```python
from build123d import *

# Parameters (mm, degrees)
SKETCH1_W           = 31.25
SKETCH1_H           = 36.32
SKETCH1_R           = 1.5
BOSS_EXTRUDE2_DEPTH = 2
FILLET1_R           = 2
BOSS_EXTRUDE3_DEPTH = 6


with BuildPart() as part:
    # Sketch1 → Boss-Extrude2 (new body)
    with BuildSketch(Plane(origin=(0, 0, 0), x_dir=(1, 0, 0), z_dir=(0, 1, 0))):
        with Locations((-0.273367395, -0.136683698)):
            Rectangle(SKETCH1_W, SKETCH1_H)
        with Locations((-0.273367395, 14.023316302)):
            Circle(SKETCH1_R, mode=Mode.SUBTRACT)
        with Locations((-11.898367395, -0.136683698)):
            Circle(SKETCH1_R, mode=Mode.SUBTRACT)
        with Locations((-0.273367395, -14.296683698)):
            Circle(SKETCH1_R, mode=Mode.SUBTRACT)
        with Locations((11.351632605, -0.136683698)):
            Circle(SKETCH1_R, mode=Mode.SUBTRACT)
    extrude(amount=BOSS_EXTRUDE2_DEPTH)

    # Fillet1
    fillet1_edges = [part.edges().sort_by_distance(p)[0] for p in [
        (15.351632605, 1, 18.296683698),
        (-15.898367395, 1, 18.296683698),
        (-15.898367395, 1, -18.023316302),
        (15.351632605, 1, -18.023316302),
    ]]
    fillet(fillet1_edges, radius=FILLET1_R)

    # Sketch3 → Boss-Extrude3 (add)
    with BuildSketch(Plane(origin=(0, 2, 0), x_dir=(1, 0, 0), z_dir=(0, 1, 0))):
        with BuildLine():
            Line((13.351632605, 19.523316302), (-13.898367395, 19.523316302))
            ThreePointArc((-13.898367395, 19.523316302), (-16.373241129, 18.498190037), (-17.398367395, 16.023316302))
            Line((-17.398367395, 16.023316302), (-17.398367395, -16.296683698))
            ThreePointArc((-17.398367395, -16.296683698), (-16.373241129, -18.771557432), (-13.898367395, -19.796683698))
            Line((-13.898367395, -19.796683698), (13.351632605, -19.796683698))
            ThreePointArc((13.351632605, -19.796683698), (15.826506339, -18.771557432), (16.851632605, -16.296683698))
            Line((16.851632605, -16.296683698), (16.851632605, 16.023316302))
            ThreePointArc((16.851632605, 16.023316302), (15.826506339, 18.498190037), (13.351632605, 19.523316302))
        make_face()
        with BuildLine():
            Line((13.351632605, 18.023316302), (-13.898367395, 18.023316302))
            ThreePointArc((-13.898367395, 18.023316302), (-15.312580957, 17.437529865), (-15.898367395, 16.023316302))
            Line((-15.898367395, 16.023316302), (-15.898367395, -16.296683698))
            ThreePointArc((-15.898367395, -16.296683698), (-15.312580957, -17.71089726), (-13.898367395, -18.296683698))
            Line((-13.898367395, -18.296683698), (13.351632605, -18.296683698))
            ThreePointArc((13.351632605, -18.296683698), (14.765846167, -17.71089726), (15.351632605, -16.296683698))
            Line((15.351632605, -16.296683698), (15.351632605, 16.023316302))
            ThreePointArc((15.351632605, 16.023316302), (14.765846167, 17.437529865), (13.351632605, 18.023316302))
        make_face(mode=Mode.SUBTRACT)
    extrude(amount=-BOSS_EXTRUDE3_DEPTH)


solid = part.part
```
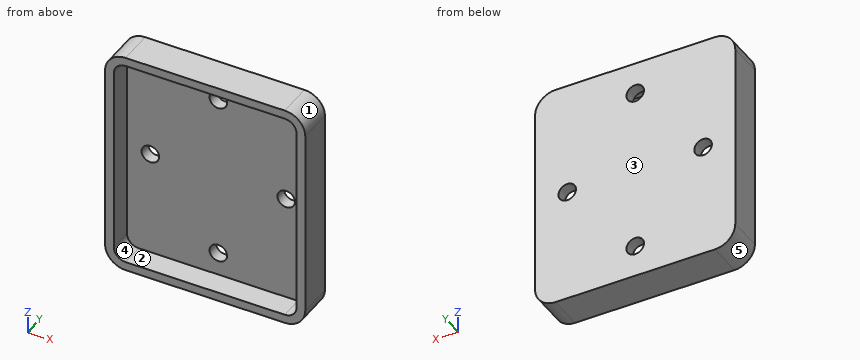
Geometry check sheet. Reference: the model listing, model coordinates, mm. Face numbers are marked on the shaded views. A direction names the side the tool comes from. Coordinates: 2 decimals unless noted, no trailing zeros. Order: outer loops, then holes, each group sorted by start corner. A loop starts at its lowest first (then second) coordinate and runs counter-clockwise, first axis right, second up. Notation, with made-up numbers: (66.5, 5.5) - (92.5, 5.5) arc R34 cw to (92.5, 42.5) - close; hole circle Ø6 at (87.5, -36). An arc over 180 degrees is marked (long way). Answer in a Markdown table with one row per item. Add a question column.
1. Draft check along Z on the marked faces 3, 4 and 5. Enter one of: +Z half, -Z half, draft (parallel to the pull), parting line (faces both ways), or undercut.
2. Access from +Z, -Z, +X, -X, +Y, -Y to the whole of each face (thin tool, end or side, straight path). Record for the marked faces 1 and 2.
3. Section check D-D (x = 0.5). Enter the section's corners in (y, z).
4. Section check C-C (x = -8.5). Enter the section's corners in (y, z), plus the area to 3 significant figures.
5. Section check A-A (y = -0.5). Enter the section's corners in (x, z), plus the area to 3 significant figures.
6. Material ranges on L1, parallel to Z at x = 12, y = -1.6; L2, parallel to X at y = -2.8, z = -16; L3, parallel to Z at x = -12, y = 0.7, recorded low to high. Write a range as [from, to].
7. Section check B-B (z = -13). Enter the section's corners in (x, y), plus the area to 3 significant figures.
8. Gauge pin test, flat end, axial feed: pin 1 Ø6 at (x, z) = (-4.5, -8.5) entering from -Y. Record the tip position at first contact, or that the pin passes through.
Data:
| question | item | result |
|---|---|---|
| 1 | face 3 | draft |
| 1 | face 4 | undercut |
| 1 | face 5 | -Z half |
| 2 | face 1 | +Z, +X, +Y, -Y |
| 2 | face 2 | -Y |
| 3 | outline | (-4, -19.52) - (2, -19.52) - (2, -15.31) - (0, -15.31) - (0, -18.02) - (-4, -18.02) - close; (-4, 18.3) - (0, 18.3) - (0, 15.58) - (2, 15.58) - (2, 19.8) - (-4, 19.8) - close; (0, -12.74) - (2, -12.74) - (2, 13.01) - (0, 13.01) - close |
| 4 | outline | (-4, -19.52) - (2, -19.52) - (2, 19.8) - (-4, 19.8) - (-4, 18.3) - (0, 18.3) - (0, -18.02) - (-4, -18.02) - close |
| 4 | area | 90.6 mm² |
| 5 | outline | (-17.4, -16.02) arc R3.5 ccw to (-13.9, -19.52) - (13.35, -19.52) arc R3.5 ccw to (16.85, -16.02) - (16.85, 16.3) arc R3.5 ccw to (13.35, 19.8) - (-13.9, 19.8) arc R3.5 ccw to (-17.4, 16.3) - close; hole (-15.9, -16.02) arc R2 ccw to (-13.9, -18.02) - (13.35, -18.02) arc R2 ccw to (15.35, -16.02) - (15.35, 16.3) arc R2 ccw to (13.35, 18.3) - (-13.9, 18.3) arc R2 ccw to (-15.9, 16.3) - close |
| 5 | area | 205 mm² |
| 6 | L1 | z = [-19.52, -18.02], [18.3, 19.8] |
| 6 | L2 | x = [-17.4, -15.9], [15.35, 16.85] |
| 6 | L3 | z = [-19.52, -1.36], [1.63, 19.8] |
| 7 | outline | (-17.4, -4) - (-15.9, -4) - (-15.9, 0) - (-1.37, 0) - (-1.37, 2) - (-17.4, 2) - close; (0.82, 0) - (15.35, 0) - (15.35, -4) - (16.85, -4) - (16.85, 2) - (0.82, 2) - close |
| 7 | area | 76.1 mm² |
| 8 | pin 1 | stops at y = 0 |
